Check sheet for the modelled part. Datum: model origin and axes. Units: mm. Coordinates: 2 decimals unless noted, no trailing zeros. Loops run counter-clockwise (first coordinate to the right, second up) from the corner with the lowest first, then second, coordinate; pieces in that order, holes last.
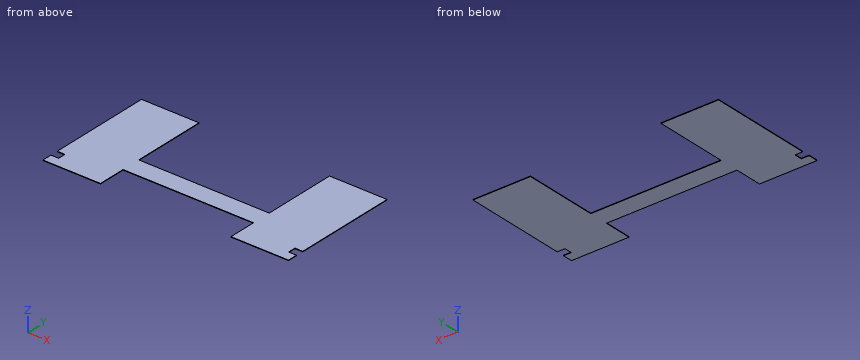
```python
from build123d import *

# Parameters (mm, degrees)
BOSS_EXTRUDE1_DEPTH = 1.5875
SKETCH2_W           = 25.4
SKETCH2_H           = 25.4
CUT_EXTRUDE1_DEPTH  = 2.5875
SKETCH3_W           = 25.4
SKETCH3_H           = 25.4
CUT_EXTRUDE2_DEPTH  = 2.5875


with BuildPart() as part:
    # Sketch1 → Boss-Extrude1 (new body)
    with BuildSketch(Plane.XY):
        Polygon((-400.05, 241.3), (-400.05, -153.162), (-212.725, -153.162), (-212.725, -62.738), (212.725, -62.738), (212.725, -153.162), (400.05, -153.162), (400.05, 241.3), (212.725, 241.3), (212.725, 0), (-212.725, 0), (-212.725, 241.3), align=None)
    extrude(amount=BOSS_EXTRUDE1_DEPTH)

    # Sketch2 → Cut-Extrude1 (cut, through all)
    with BuildSketch(Plane(origin=(0, 0, 0), x_dir=(-1, 0, 0), z_dir=(0, 0, -1))):
        with Locations((-387.35, -108.712)):
            Rectangle(SKETCH2_W, SKETCH2_H)
    extrude(amount=-CUT_EXTRUDE1_DEPTH, mode=Mode.SUBTRACT)

    # Sketch3 → Cut-Extrude2 (cut, through all)
    with BuildSketch(Plane(origin=(0, 0, 0), x_dir=(-1, 0, 0), z_dir=(0, 0, -1))):
        with Locations((387.35, -108.712)):
            Rectangle(SKETCH3_W, SKETCH3_H)
    extrude(amount=-CUT_EXTRUDE2_DEPTH, mode=Mode.SUBTRACT)


solid = part.part
```
1) Depth check by flat-ended pin: pin 1 (0.8 mm diameter, centred on y = -114.5, z = 0.5, fed in from +X); pin 2 (0.8 mm diameter, centred on y = -111.5, z = 0.5, fed in from -X); pin 3 (0.5 mm diameter, centred on x = 58.5, z = 0.5, fed in from -Y). Enter the tip coordinate at first touch or a pass-through.
Answer sheet:
pin 1: stops at x = 374.65
pin 2: stops at x = -374.65
pin 3: stops at y = -62.74
2) Section check C-C on x = 82.5. Enter the section's corners in (y, z), plus the area to 3 significant figures.
Answer sheet:
outline: (-62.74, 0) - (0, 0) - (0, 1.59) - (-62.74, 1.59) - close
area: 99.6 mm2
3) Section check B-B on z = 0.95. Enter the section's corners in (x, y) (3 decimals), plus the area to 3 significant figures.
Answer sheet:
outline: (-400.05, -153.162) - (-212.725, -153.162) - (-212.725, -62.738) - (212.725, -62.738) - (212.725, -153.162) - (400.05, -153.162) - (400.05, -121.412) - (374.65, -121.412) - (374.65, -96.012) - (400.05, -96.012) - (400.05, 241.3) - (212.725, 241.3) - (212.725, 0) - (-212.725, 0) - (-212.725, 241.3) - (-400.05, 241.3) - (-400.05, -96.012) - (-374.65, -96.012) - (-374.65, -121.412) - (-400.05, -121.412) - close
area: 173,000 mm2
4) Scan lines: line 1 (X direction, y = -66.5, z = 1.1) (3 decimals); line 2 (Y direction, x = 108, z = 0.85). Record each from-to range of solid material in increasing order.
Answer sheet:
line 1: x = -400.05 to -212.725, 212.725 to 400.05
line 2: y = -62.74 to 0
